Geometry: final body of the model. Coordinates: model frame, mm. Face numbers are marked on the shaded views. A direction names the side the tool comes from. Give positions to 0.01 mm unless a question says otherwise; leave off trailing zeros. Order: outer loops, then holes, each group sorted by start corner. A loop starts at its lowest first (then second) coordinate and runs counter-clockwise, first axis right, second up. Notation, with made-up numbers: (39, -14.5) -> (67, -14.5) arc R6 ccw to (67, -6.5) -> close; hole circle Ø6 at (82, 31.5). An arc over 180 degrees is marked (long way). One line per question, with ' | ' between items.
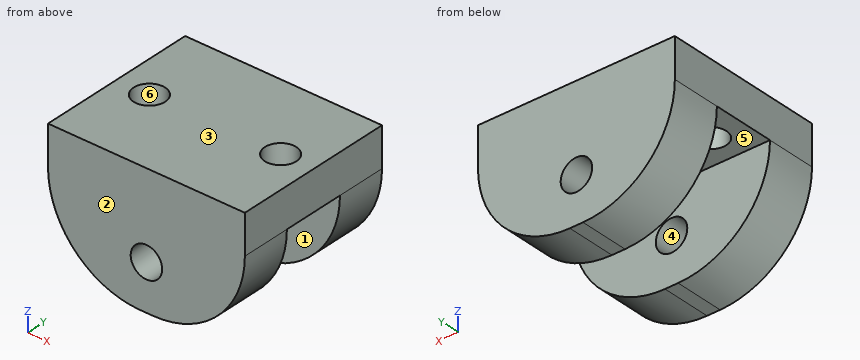
from build123d import *

# Parameters (mm, degrees)
BOSS_EXTRUDE1_DEPTH = 75
SKETCH2_R           = 6
CUT_EXTRUDE1_DEPTH  = 110.402925007
SKETCH3_R           = 6
CUT_EXTRUDE2_DEPTH  = 110.402925007
FILLET1_R           = 35


with BuildPart() as part:
    # Sketch1 → Boss-Extrude1 (new body)
    with BuildSketch(Plane(origin=(0, 0, 0), x_dir=(0, 0, -1), z_dir=(1, 0, 0))):
        Polygon((50, 62), (50, 43), (15, 43), (15, 19), (50, 19), (50, 0), (0, 0), (0, 62), align=None)
    extrude(amount=BOSS_EXTRUDE1_DEPTH)

    # Sketch2 → Cut-Extrude1 (cut, through all)
    with BuildSketch(Plane.XY):
        with Locations((62.5, 31)):
            Circle(SKETCH2_R)
        with Locations((12.5, 31)):
            Circle(SKETCH2_R)
    extrude(amount=-CUT_EXTRUDE1_DEPTH, mode=Mode.SUBTRACT)

    # Sketch3 → Cut-Extrude2 (cut, through all)
    with BuildSketch(Plane(origin=(0, 62, 0), x_dir=(1, 0, 0), z_dir=(0, 1, 0))):
        with Locations(Location((37.5, 32.5, 0), (0, 0, 270))):
            Circle(SKETCH3_R)
    extrude(amount=-CUT_EXTRUDE2_DEPTH, mode=Mode.SUBTRACT)

    # Fillet1
    fillet1_edges = [part.edges().sort_by_distance(p)[0] for p in [
        (75, 9.5, -50),
        (0, 9.5, -50),
        (0, 52.5, -50),
        (75, 52.5, -50),
    ]]
    fillet(fillet1_edges, radius=FILLET1_R)


solid = part.part
1) Contact query for flat-ended pins moving along their axis: pin 1 Ø8 at (y, z) = (15.5, -27) entering from +X; pin 2 Ø6 at (y, z) = (17.5, -42.5) entering from -X (3 decimals); pin 3 Ø19 at (x, y) = (53.5, 36.5) entering from -Z. Output: stop coordinate, or through.
Check result:
pin 1: stops at x = 74.07 | pin 2: stops at x = 10.005 | pin 3: stops at z = -49.38
2) Set-up query: the marked faces 1 and 2. Return all of +Z, -Z, +X, -X, +Y, -Y with unobstructed straight access to the full face (end or side cutting, diameter ignored); none if empty.
Check result:
face 1: -Z, +X, -X | face 2: +Z, -Z, +X, -X, -Y
3) Section D-D on z = -30. Return loops of the section in (x, y).
Check result:
outline: (3.38, 0) -> (32.05, 0) -> (32.05, 19) -> (3.38, 19) -> close; (3.38, 43) -> (32.05, 43) -> (32.05, 62) -> (3.38, 62) -> close; (42.95, 0) -> (71.62, 0) -> (71.62, 19) -> (42.95, 19) -> close; (42.95, 43) -> (71.62, 43) -> (71.62, 62) -> (42.95, 62) -> close
4) Material intervals for probe 1 along Y at (x, z) = (59, -16); probe 2 along Y at (x, z) = (12, -10); probe 3 along Z at (x, y) = (37, 57), sorted ascending. Write a range as from..to.
Check result:
probe 1: y = 0..19, 43..62 | probe 2: y = 0..25.02, 36.98..62 | probe 3: z = -50..-38.48, -26.52..0
5) Section C-C on y = 17. Return loops of the section in (x, z).
Check result:
outline: (0, -15) arc R35 ccw to (35, -50) -> (40, -50) arc R35 ccw to (75, -15) -> (75, 0) -> (0, 0) -> close; hole circle Ø12 at (37.5, -32.5)
6) Section A-A on y = 31. Return loops of the section in (x, z), plus the area to 3 significant figures.
Check result:
outline: (0, -15) -> (6.5, -15) -> (6.5, 0) -> (0, 0) -> close; (18.5, -15) -> (56.5, -15) -> (56.5, 0) -> (18.5, 0) -> close; (68.5, -15) -> (75, -15) -> (75, 0) -> (68.5, 0) -> close | area: 765 mm^2
7) Pull-direction query (Z, two-part tool) for the marked faces 3, 4, 5 and 6; classes: +Z half, -Z half, draft (parallel to the pull), parting line (faces both ways), or undercut.
Check result:
face 3: +Z half | face 4: undercut | face 5: -Z half | face 6: draft
8) Section B-B on x = 12.5. Return loops of the section in (y, z), plus the area to 3 significant figures.
Check result:
outline: (0, -41.81) -> (19, -41.81) -> (19, -15) -> (25, -15) -> (25, 0) -> (0, 0) -> close; (37, -15) -> (43, -15) -> (43, -41.81) -> (62, -41.81) -> (62, 0) -> (37, 0) -> close | area: 1,770 mm^2
